Could you check a few things on this drawing? It's one solid part, dimensions in mm from its lowest x, y, z. A direction names the side the tool comes from. Give positions to 0.01 mm unless a question says otherwise; leave off trailing zeros. Write each loop counter-clockwise with the first axis right and the second up, starting at its lowest first coordinate (ties: lowest second). Pieces come first, ordered by that corner, then holes. Notation, with made-up numbers: M 66,-19 L 88,-19 A25 ccw 88,-4 Z; hole C -5.5,-28.75 d5. An arc over 180 degrees is marked long. Answer as CSV lines item,"result". Start each with the question number.
Q1. On a 3-axis mill with a long thin cutter (end or side, diameter ignored), from which of +Z, -Z, +X, -X, +Y, -Y can I reach the whole of each face in a straight line? I mean the marked faces 1, 2 and 3. Say none if no direction works.
Q2. Suppose I cut it at A-A (y = 5.75). Write out the boundary of the cut face in (x, z).
Q3. Thinking about a two-plate mould opening in X: for the marked faces 4, 5 and 6, which applies, +X half, -X half, draft (parallel to the pull), parting line (faces both ways), or undercut?
Q4. If I drill on line 1 along Y through (x, z) = (1.15, 0.8); line 2 along X through (y, z) = (10.25, 2.35); line 3 along Y through (x, z) = (2.8, 3.45), over which ranges is the centre line in solid material (lowest first)?
Q5. For pin 1 (3 mm diameter, centred on x = 1, y = 4.5, fed in from +Z); pin 2 (1 mm diameter, centred on x = 4.5, y = 9, fed in from -Z), each with a flat end and sliding along its axis, tell me the tip position at first contact or that it passes through.
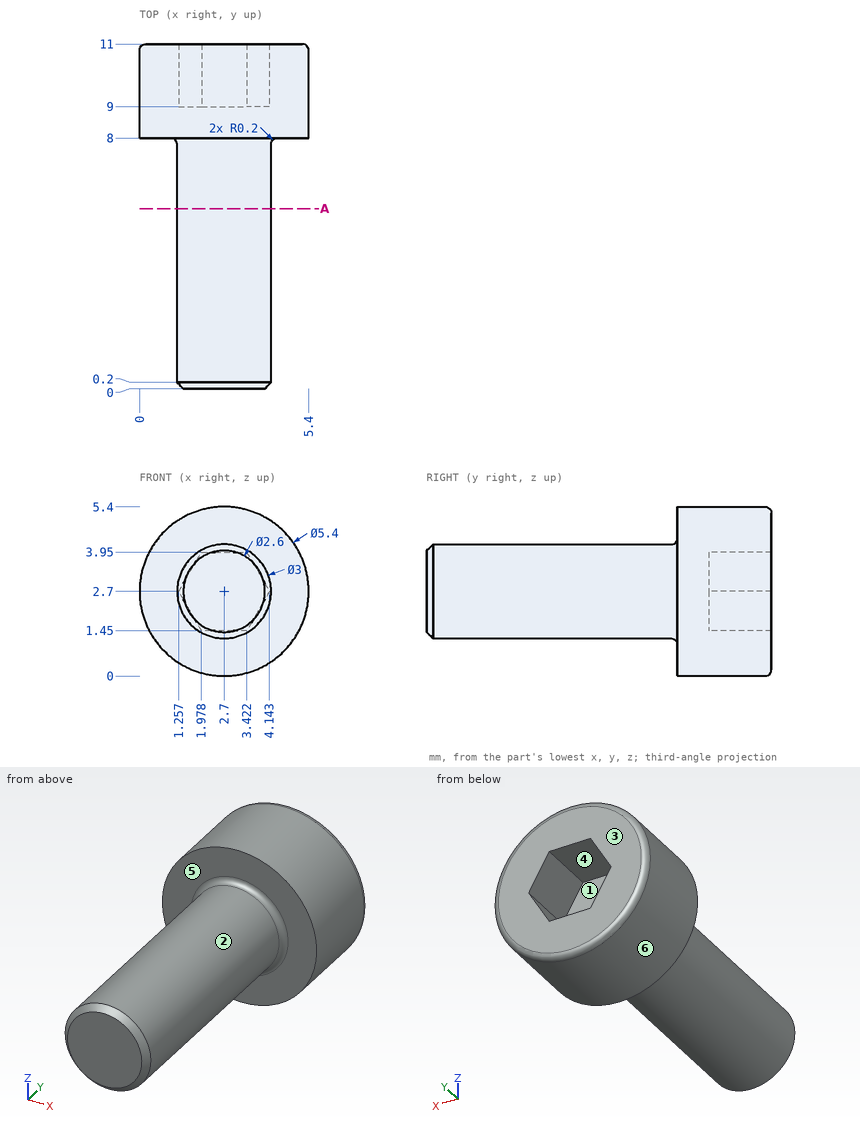
Resolved:
1,face 1,"+Y"
1,face 2,"-Y"
1,face 3,"+Z, -Z, +X, -X, +Y"
2,outline,"C 2.7,2.7 d3"
3,face 4,"undercut"
3,face 5,"draft"
3,face 6,"parting line"
4,line 1,"8 to 11"
4,line 2,"0.02 to 1.46, 3.94 to 5.38"
4,line 3,"0 to 9"
5,pin 1,"z = 4.19"
5,pin 2,"z = 0.33"
